Geometry check sheet. Reference: the model listing, model coordinates, mm. A direction names the side the tool comes from. Coordinates: 2 decimals unless noted, no trailing zeros. Loops run counter-clockwise (first coordinate to the right, second up) from the corner with the lowest first, then second, coordinate; pieces in that order, holes last.
Autodesk Inventor part; units mm, degrees
ref_plane "YZ Plane" through (0, 0, 0) normal (1, 0, 0) x (0, 1, 0)
ref_plane "XZ Plane" through (0, 0, 0) normal (0, 1, 0) x (-1, 0, 0)
ref_plane "XY Plane" through (0, 0, 0) normal (0, 0, 1) x (1, 0, 0)
sketch "Sketch1" plane through (0, 0, 0) normal (0, 1, 0) x (-1, 0, 0)
  line L0 (0, 0) -> (9.5, 0)
  line L1 (9.5, 0) -> (9.5, -64)
  line L2 (9.5, -64) -> (0, -64)
  line L3 (0, -64) -> (0, 0)
  circle A0 centre (3.7, -11.5) radius 2.25
  circle A1 centre (3.7, -59.5) radius 2.25
  line L4 (3.7, -11.5) -> (3.7, -59.5) construction
  dimension "d1" = 9.5
  dimension "d2" = 64
  dimension "d3" = 4.5
  dimension "d4" = 48
  dimension "d6" = 3.7
  dimension "d17" = 4.5
extrude "Extrusion1" add sketch "Sketch1" along normal blind 12
sketch "Sketch2" plane through (-9.5, 0, 0) normal (0, 0, 1) x (1, 0, 0)
  line L0 (9.5, 12) -> (0, 12)
  line L1 (3, 12) -> (8.4, 12)
  line L2 (8.4, 12) -> (8.4, 10.8)
  line L3 (8.4, 10.8) -> (3, 10.8)
  line L4 (3, 10.8) -> (3, 12)
  line L5 (9.5, 0) -> (9.5, 12)
  line L6 (3.55, 0) -> (8.05, 0)
  line L7 (3.55, 12) -> (8.05, 12)
  line L8 (9.5, 0) -> (9.5, 12)
  line L9 (9.5, 0) -> (9.5, 12)
  line L10 (3.55, 12) -> (8.05, 12)
  line L11 (3.55, 12) -> (3.55, 0)
  line L12 (3.55, 12) -> (8.05, 12)
  line L13 (3.55, 0) -> (8.05, 0)
  line L14 (3.55, 12) -> (8.05, 12)
  line L15 (3.55, 0) -> (8.05, 0)
  line L16 (3.55, 12) -> (8.05, 12)
  line L17 (3.55, 0) -> (8.05, 0)
  dimension "d9" = 1.1
  dimension "d10" = 5.4
  dimension "d11" = 1.2
  dimension "d76" = 12
extrude "Extrusion2" cut sketch "Sketch2" against normal up to next
sketch "Sketch3" plane through (0, 0, 0) normal (0, -1, 0) x (1, 0, 0)
  circle A0 centre (-3.7, -11.5) radius 2.25
  circle A1 centre (-3.7, -11.5) radius 3.75
  circle A2 centre (-3.7, -59.5) radius 2.25
  circle A3 centre (-3.7, -59.5) radius 3.75
  point P0 (0, 0)
  dimension "d14" = 7.5
extrude "Extrusion3" cut sketch "Sketch3" against normal blind 3
fillet "Fillet1" radius 1 4 edges at (0, 1.5, -58.8897) (0, 1.5, -60.1103) (0, 1.5, -10.8897) (0, 1.5, -12.1103)
fillet "Fillet2" radius 4 2 edges at (-9.5, 6, -64) (-9.5, 6, 0)
sketch "Sketch15" plane through (0, 0, 0) normal (0, -1, 0) x (1, 0, 0)
  line L0 (0, 0) -> (0, -7.592)
  line L1 (-9.5, -32) -> (-9.5, -21)
  line L2 (-9.5, -21) -> (0, -21)
  line L3 (0, -21) -> (0, -43)
  line L4 (0, -43) -> (-9.5, -43)
  line L5 (-9.5, -43) -> (-9.5, -32)
  dimension "d79" = 11
  dimension "d80" = 22
extrude "Extrusion15" add sketch "Sketch15" along normal blind 15
sketch "Sketch21" plane through (0, -15, 0) normal (0, -1, 0) x (1, 0, 0)
  line L0 (-9.5, -43) -> (-19.5, -43)
  line L1 (-19.5, -43) -> (-19.5, -33)
  line L2 (-19.5, -33) -> (20.5, -33)
  line L3 (20.5, -33) -> (20.5, -43)
  line L4 (20.5, -43) -> (-9.5, -43)
  point P0 (0, 0)
  dimension "d93" = 10
  dimension "d94" = 10
  dimension "d95" = 40
  dimension "d96" = 10
extrude "Extrusion17" add sketch "Sketch21" along normal blind 10
sketch "Sketch27" plane through (0, -25, 0) normal (0, -1, 0) x (1, 0, 0)
  line L0 (-19.5, -33) -> (-19.5, -43)
  line L1 (-19.5, -43) -> (20.5, -43)
  line L2 (-19.5, -33) -> (20.5, -33)
  line L3 (20.5, -33) -> (20.5, -43)
  line L4 (20.5, -43) -> (-19.5, -43)
  line L5 (-19.5, -43) -> (-19.5, -33)
  point P0 (0, 0)
sketch "Sketch28" plane through (20.5, -15, -33) normal (1, 0, 0) x (0, 0, -1)
  line L0 (10, -10) -> (0, -10)
  arc A0 (5, -80) -> (5, -10) centre (-43.734, -45) ccw
  point P0 (-33, 15)
  dimension "d101" = 70
  dimension "d102" = 60
sweep "Sweep1" add profiles "Sketch27" path "Sketch28" path curves A0
properties part number "Front"
1) Section check A-A on x = -3.7. Record the cut outline in (y, z), and give its area (3 significant figures).
Data:
outline: (-99.74, -39.6) arc R64.13 ccw to (-25, -43) - (0, -43) - (0, -55.75) - (3, -55.75) - (3, -57.25) - (10.8, -57.25) - (10.8, -13.75) - (3, -13.75) - (3, -15.25) - (0, -15.25) - (0, -21) - (-15, -21) - (-15, -33) - (-25, -33) arc R56.01 cw to (-90.26, -36.4) - close; (0, -64) - (10.8, -64) - (10.8, -61.75) - (3, -61.75) - (3, -63.25) - (0, -63.25) - close; (0, -7.75) - (3, -7.75) - (3, -9.25) - (10.8, -9.25) - (10.8, 0) - (0, 0) - close
area: 1,610 mm2
2) Section check B-B on z = -18. Record the cut outline in (x, y).
Data:
outline: (-9.5, 0) - (0, 0) - (0, 12) - (-1.1, 12) - (-1.1, 10.8) - (-6.5, 10.8) - (-6.5, 12) - (-9.5, 12) - close
3) Mould release check, pull along Z, two halves, no side actions. Record for faces 6 (the flat face through (-3, 6, -64)), 7 (the flat face through (-9.5, 1, -32)), 8 (the flat face through (-1, 3, -11)), 9 (the cylindrical face through (-4.738, 6.845, -57.504)): +Z half, -Z half, draft (parallel to the pull), parting line (faces both ways), or undercut.
Data:
face 6: -Z half
face 7: draft
face 8: undercut
face 9: undercut
4) Section check C-C on z = -11.5. Record the cut outline in (x, y), and give its area (3 significant figures).
Data:
outline: (-9.5, 0) - (-7.45, 0) - (-7.45, 3) - (-5.95, 3) - (-5.95, 10.8) - (-6.5, 10.8) - (-6.5, 12) - (-9.5, 12) - close; (-1.45, 3) - (0, 3) - (0, 12) - (-1.1, 12) - (-1.1, 10.8) - (-1.45, 10.8) - close
area: 50.1 mm2
5) Section check D-D on x = 4. Record the cut outline in (y, z), and give its area (3 significant figures).
Data:
outline: (-99.74, -39.6) arc R64.13 ccw to (-25, -43) - (-15, -43) - (-15, -33) - (-25, -33) arc R56.01 cw to (-90.26, -36.4) - close
area: 707 mm2
6) Depth check by flat-ended pin: pin 1 (0.6 mm diameter, centred on y = 11.5, z = -42, fed in from -X); pin 2 (5 mm diameter, centred on x = 9, z = -37.5, fed in from +Y); pin 3 (5 mm diameter, centred on x = -3.5, z = -10, fed in from -Y). Enter the tip coordinate at first touch or a pass-through.
Data:
pin 1: stops at x = -9.5
pin 2: stops at y = -15
pin 3: stops at y = 0
7) Material ranges on probe 1 along X at (y, z) = (7, -11.5); probe 2 along Z at (x, y) = (-3, 1); probe 3 along X at (y, z) = (5.5, -28), recorded low to high.
Data:
probe 1: x = -9.5 to -5.95, -1.45 to 0
probe 2: z = -64 to -63.18, -55.82 to -15.18, -7.82 to 0
probe 3: x = -9.5 to 0
8) Access from +Z, -Z, +X, -X, +Y, -Y to the whole of each face (thin tool, end or side, straight path). Record for faces 1 (the cylindrical face through (-7.45, 1.48, -59.39)), 2 (the flat face through (0, 1, -32)), 3 (the flat face through (-5, 0, -51)), 4 (the flat face through (-6, 0, -8)), 5 (the flat face through (-4, 10.8, -32)).
Data:
face 1: -Y
face 2: +Z, -Z, +X, +Y
face 3: -Z, +X, -X
face 4: +Z, +X, -X, -Y
face 5: +Z, -Z, +Y
